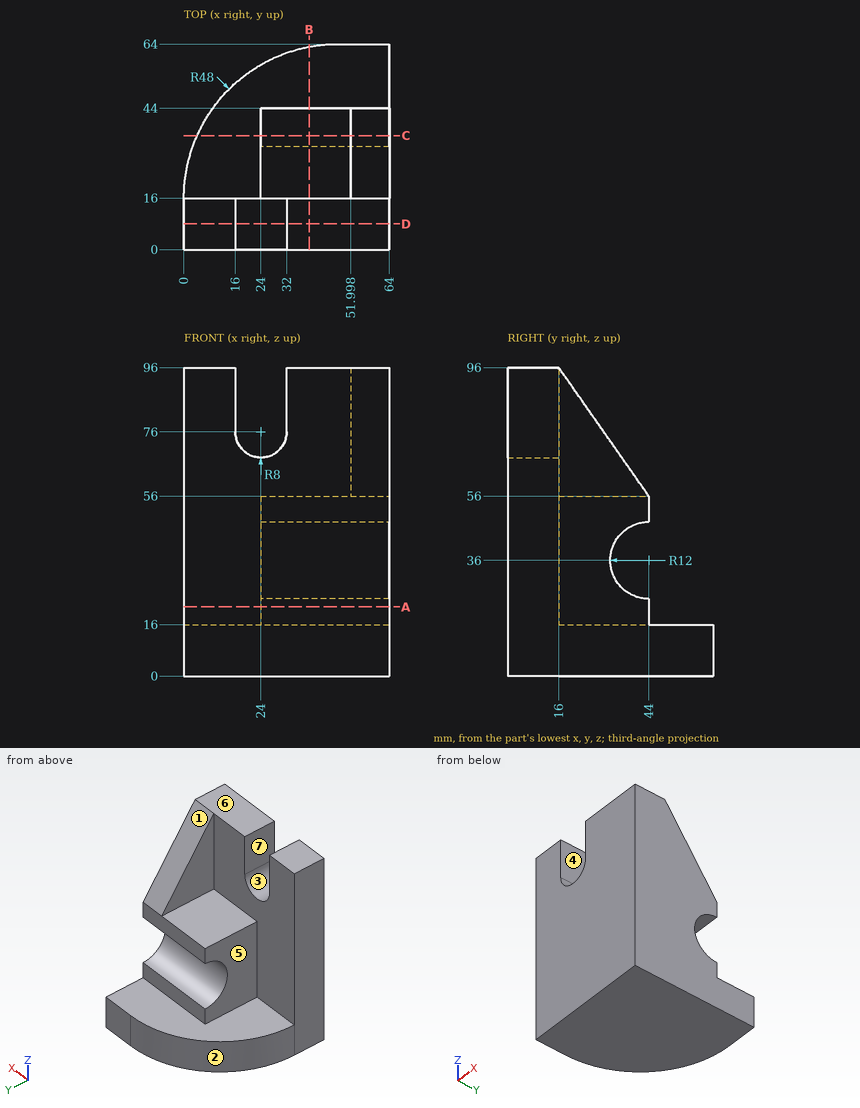
The figure shows three views and two pictorial views of one solid part (mm, origin at its lowest corner). Answer the questions. A direction names the side the tool comes from. Coordinates: 2 decimals unless noted, no trailing zeros. Loops run counter-clockwise (first coordinate to the right, second up) from the corner with the lowest first, then second, coordinate; pieces in that order, holes last. Notation, with made-up numbers: (-17, -38) -> (2, -38) arc R20 cw to (2, -14) -> close; hole circle Ø11 at (-15.5, -4). An arc over 180 degrees is marked (long way). Return JSON: item names as keys, results as strings. Group by question number.
(1) A cutting plane is placed at D-D on y = 8. Write down the section's boundary in (x, z), and give its area (3 significant figures).
(2) A cutting plane is placed at B-B on x = 39. Write down the section's boundary in (y, z).
(3) A cutting plane is placed at A-A on z = 21.5. Write down the section's boundary in (x, y), and give its area (3 significant figures).
(4) Which of the six approach directions +Z, -Z, +X, -X, +Y, -Y give full straight-line access (tool end or side, diameter ignored) to the marked faces 5, 6 and 7?
(5) A cutting plane is placed at C-C on y = 35.5. Write down the section's boundary in (x, z), and give its area (3 significant figures).
(6) Find the intervals of material crossed by probe 1 along Y at (x, z) = (57, 20); probe 2 along Z at (x, y) = (46.5, 45.5); probe 3 along Z at (x, y) = (32.5, 33) (1 decimal), in increasing order. Write a range as from..to.
(7) Determine the mould class of the marked faces 1, 2, 3 and 4 for opening direction X: released by +X, released by -X, zero draft, split by the parting line, or undercut.
(8) Given pin 1 Ø1 at (x, z) = (14.5, 23) entering from +Y; pin 2 Ø9 at (x, z) = (44, 18.5) entering from +Y; pin 3 Ø9 at (x, z) = (46.5, 51) entering from +Y, each flat-ended and moving along its own axis, determine where each tip first touches the part or whether it passes through.
The answers:
{
 "1": {"outline": "(0, 0) -> (64, 0) -> (64, 96) -> (32, 96) -> (32, 76) arc R8 cw to (16, 76) -> (16, 96) -> (0, 96) -> close", "area": "5,720 mm^2"},
 "2": {"outline": "(0, 0) -> (63.15, 0) -> (63.15, 16) -> (44, 16) -> (44, 24) arc R12 cw to (44, 48) -> (44, 56) -> (16, 56) -> (16, 96) -> (0, 96) -> close"},
 "3": {"outline": "(0, 0) -> (64, 0) -> (64, 44) -> (24, 44) -> (24, 16) -> (0, 16) -> close", "area": "2,140 mm^2"},
 "4": {"face 5": "+Z, -X, +Y", "face 6": "+Z, +X, -X, +Y, -Y", "face 7": "+Z, +Y, -Y"},
 "5": {"outline": "(4.14, 0) -> (64, 0) -> (64, 27.53) -> (24, 27.53) -> (24, 16) -> (4.14, 16) -> close; (24, 44.47) -> (64, 44.47) -> (64, 68.14) -> (52, 68.14) -> (52, 56) -> (24, 56) -> close", "area": "2,030 mm^2"},
 "6": {"probe 1": "y = 0..44", "probe 2": "z = 0..16", "probe 3": "z = 0..31.2, 40.8..56"},
 "7": {"face 1": "zero draft", "face 2": "released by -X", "face 3": "undercut", "face 4": "undercut"},
 "8": {"pin 1": "stops at y = 16", "pin 2": "stops at y = 64", "pin 3": "stops at y = 44"}
}
